Geometry: final body of the model. Coordinates: model frame, mm. A direction names the side the tool comes from. Give positions to 0.01 mm unless a question says otherwise; leave off trailing zeros. Write each loop counter-clockwise with the first axis right and the second up, starting at its lowest first coordinate (ties: lowest second). Pieces come first, ordered by that corner, then holes.
Q1. Reachability of faces 4 (the face through (-3, 24.019, 2)), 5 (the face through (-39, 16.519, 2)), 6 (the face through (-21, 7.519, 2)), 7 (the face through (-39, 24.019, 2)) from +Z, -Z, +X, -X, +Y, -Y: full face, straight path, thin tool, end or side. Return the list, or none.
Q2. Cut plane A-A on y = 5.5. Return the cut outline in (x, z), plus the area to 3 significant figures.
Q3. Cut plane B-B on x = -37.5. Return the cut outline in (y, z), plus the area to 3 significant figures.
Q4. Draft query along X for faces 1 (the face through (-41.901, 25, 2)), 2 (the face through (-29, 2.519, 2)), 3 (the face through (-16.401, 5, 2)). Return one class per face: pulls with the +X half, pulls with the -X half, needs draft (parallel to the pull), parting line crosses it, or undercut.
Q5. Line query: L1, parallel to Y at x = -39.5, z = 3; L2, parallel to X at y = 11.75, z = 3.65; L3, parallel to X at y = 23.75, z = 0.55. Output: solid intervals per line, ascending.
Q6. Cut plane C-C on z = 3.9. Return the cut outline in (x, y).
Q7. Cut plane D-D on x = -20. Return the cut outline in (y, z).
Q8. Pin query (flat end, axial travel): pin 1 (2 mm diameter, centred on y = 7.5, z = 2.5, fed in from -X); pin 2 (1.5 mm diameter, centred on x = -39.5, z = 2, fed in from -Y); pin 3 (2.5 mm diameter, centred on y = 21.5, z = 1.5, fed in from -X). Return the tip coordinate at first contact, or that it passes through.
```python
from build123d import *

# Parameters (mm, degrees)
BOSS_EXTRU_1_DEPTH = 5


with BuildPart() as part:
    # Esquisse1 → Boss.-Extru.1 (new body)
    with BuildSketch(Plane.XY):
        Polygon((-21.401470553, 26.519094535), (-21.401470553, 7.519094535), (-16.401470553, 7.519094535), (-16.401470553, 2.519094535), (-11.401470553, 2.519094535), (-11.401470553, 7.519094535), (-6.401470553, 7.519094535), (-6.401470553, 16.519094535), (-0.901470553, 16.519094535), (-0.901470553, 19.019094535), (-5.901470553, 19.019094535), (-5.901470553, 24.019094535), (-0.901470553, 24.019094535), (-0.901470553, 26.519094535), align=None)
        Polygon((-41.901470553, 16.519094535), (-36.401470553, 16.519094535), (-36.401470553, 7.519094535), (-31.401470553, 7.519094535), (-31.401470553, 2.519094535), (-26.401470553, 2.519094535), (-26.401470553, 7.519094535), (-21.401470553, 7.519094535), (-21.401470553, 26.519094535), (-41.901470553, 26.519094535), (-41.901470553, 24.019094535), (-36.901470553, 24.019094535), (-36.901470553, 19.019094535), (-41.901470553, 19.019094535), align=None)
    extrude(amount=BOSS_EXTRU_1_DEPTH)


solid = part.part
```
Data:
1. face 4: +Z, -Z, +X
1. face 5: +Z, -Z, -X, -Y
1. face 6: +Z, -Z, -Y
1. face 7: +Z, -Z, -X
2. outline: (-31.4, 0) - (-26.4, 0) - (-26.4, 5) - (-31.4, 5) - close; (-16.4, 0) - (-11.4, 0) - (-11.4, 5) - (-16.4, 5) - close
2. area: 50.0 mm2
3. outline: (16.52, 0) - (19.02, 0) - (19.02, 5) - (16.52, 5) - close; (24.02, 0) - (26.52, 0) - (26.52, 5) - (24.02, 5) - close
3. area: 25.0 mm2
4. face 1: pulls with the -X half
4. face 2: needs draft
4. face 3: undercut
5. L1: y = 16.52 to 19.02, 24.02 to 26.52
5. L2: x = -36.4 to -6.4
5. L3: x = -36.9 to -5.9
6. outline: (-41.9, 16.52) - (-36.4, 16.52) - (-36.4, 7.52) - (-31.4, 7.52) - (-31.4, 2.52) - (-26.4, 2.52) - (-26.4, 7.52) - (-16.4, 7.52) - (-16.4, 2.52) - (-11.4, 2.52) - (-11.4, 7.52) - (-6.4, 7.52) - (-6.4, 16.52) - (-0.9, 16.52) - (-0.9, 19.02) - (-5.9, 19.02) - (-5.9, 24.02) - (-0.9, 24.02) - (-0.9, 26.52) - (-41.9, 26.52) - (-41.9, 24.02) - (-36.9, 24.02) - (-36.9, 19.02) - (-41.9, 19.02) - close
7. outline: (7.52, 0) - (26.52, 0) - (26.52, 5) - (7.52, 5) - close
8. pin 1: stops at x = -36.4
8. pin 2: stops at y = 16.52
8. pin 3: stops at x = -36.9
